from build123d import *

# Parameters (mm, degrees)
BOSS_EXTRUDE1_DEPTH = 50
BOSS_EXTRUDE2_DEPTH = 10
FILLET1_R           = 15
CUT_EXTRUDE1_START  = -3
CUT_EXTRUDE1_DEPTH  = 44
FILLET2_R           = 15
BOSS_EXTRUDE3_DEPTH = 50
SKETCH5_W           = 5.55555544444444
SKETCH5_H           = 7.560737598657919
SKETCH5_W_2         = 5.5555554444444475
SKETCH5_W_3         = 5.555555444444444
CUT_EXTRUDE2_DEPTH  = 68.02665161849878
CHAMFER1_SIZE       = 2.5
CHAMFER2_SIZE       = 1


with BuildPart() as part:
    # Sketch1 → Boss-Extrude1 (new body)
    with BuildSketch(Plane(origin=(0, 0, 0), x_dir=(0, 0, -1), z_dir=(1, 0, 0))):
        Polygon((0, 0), (50.00000000000001, 0), (16.66666666666667, -40), (-8.800000000000015, -17.499999999999996), (-8.800000000000015, -12.499999999999998), (-6.200000000000014, -12.499999999999998), (-6.200000000000013, -14.499999999999998), (-2.9999999999999982, -14.499999999999998), (-2.9999999999999982, -3), (-6.200000000000013, -3), (-6.200000000000014, -4.999999999999999), (-8.800000000000015, -4.999999999999999), (-8.800000000000017, -1.08e-15), align=None)
    extrude(amount=BOSS_EXTRUDE1_DEPTH)

    # Sketch2 → Boss-Extrude2 (add)
    with BuildSketch(Plane(origin=(50, 0, 0), x_dir=(0, 0, -1), z_dir=(1, 0, 0))):
        Polygon((-8.800000000000017, -1.08e-15), (-0.800000000000016, 0), (-0.8000000000000138, -17.499999999999996), (-8.800000000000015, -17.499999999999996), align=None)
    extrude(amount=-BOSS_EXTRUDE2_DEPTH)

    # Fillet1
    fillet1_edges = [part.edges().sort_by_distance(p)[0] for p in [
        (25, -40, -16.66666666666667),
    ]]
    fillet(fillet1_edges, radius=FILLET1_R)

    # Sketch3 → Cut-Extrude1 (cut)
    with BuildSketch(Plane(origin=(50, 0, 0), x_dir=(0, 0, -1), z_dir=(1, 0, 0)).offset(CUT_EXTRUDE1_START)):
        with BuildLine():
            Line((46.000000000000014, 0), (26.501646387603547, -23.398024334875757))
            add(Edge.make_bspline(
                [(0, -15), (11.33309259276565, -40.236961436031486), (26.501646387603547, -23.398024334875757)],
                knots=[0, 0, 0, 1, 1, 1], degree=2))
            Line((0, -15), (0, 0))
            Line((0, 0), (46.000000000000014, 0))
        make_face()
    extrude(amount=-CUT_EXTRUDE1_DEPTH, mode=Mode.SUBTRACT)

    # Fillet2
    fillet2_edges = [part.edges().sort_by_distance(p)[0] for p in [
        (25, -15, 0),
    ]]
    fillet(fillet2_edges, radius=FILLET2_R)

    # Sketch4 → Boss-Extrude3 (add, through all)
    with BuildSketch(Plane(origin=(50, 0, 0), x_dir=(0, 0, -1), z_dir=(1, 0, 0))):
        Polygon((50.00000000000001, 0), (46.000000000000014, 0), (49.20092199832241, 3.841106397986878), (53.20092199832241, 3.841106397986878), align=None)
    extrude(amount=-BOSS_EXTRUDE3_DEPTH)

    # Sketch5 → Cut-Extrude2 (cut, through all)
    with BuildSketch(Plane(origin=(0, -22.622950819672138, -27.147540983606568), x_dir=(1, 0, 0), z_dir=(0, 0.6401843996644799, 0.7682212795973757))):
        Polygon((11.111111, 29.44848238456608), (11.111111, 37.009219983224), (5.555555555555555, 37.009219983224), (5.555555555555556, 29.44848238456608), align=None)
        with Locations((19.444444277777777, 33.22885118389504)):
            Rectangle(SKETCH5_W, SKETCH5_H)
        with Locations((30.555555277777778, 33.22885118389504)):
            Rectangle(SKETCH5_W_2, SKETCH5_H)
        with Locations((41.66666627777778, 33.22885118389504)):
            Rectangle(SKETCH5_W_3, SKETCH5_H)
    extrude(amount=-CUT_EXTRUDE2_DEPTH, mode=Mode.SUBTRACT)

    # Chamfer1
    chamfer1_edges = [part.edges().sort_by_distance(p)[0] for p in [
        (8.333333277777777, -3.55e-15, -46.000000000000014),
        (19.444444277777777, -3.55e-15, -46.000000000000014),
        (30.555555277777778, -3.55e-15, -46.000000000000014),
        (41.66666627777778, -3.55e-15, -46.000000000000014),
    ]]
    chamfer(chamfer1_edges, length=CHAMFER1_SIZE)

    # Chamfer2
    chamfer2_edges = [part.edges().sort_by_distance(p)[0] for p in [
        (0, -12.499999999999998, 7.500000000000014),
        (0, -13.499999999999998, 6.2000000000000135),
        (0, -14.499999999999998, 4.600000000000005),
        (0, -8.75, 2.9999999999999982),
        (0, -3, 4.600000000000005),
        (0, -3.9999999999999996, 6.2000000000000135),
        (0, -4.999999999999999, 7.500000000000014),
    ]]
    chamfer(chamfer2_edges, length=CHAMFER2_SIZE)


solid = part.part
For this review, take the finished solid that the model builds, in its own axes (mm). A direction names the side the tool comes from. Round coordinates to 2 decimals unless told otherwise and drop trailing zeros. Loops run counter-clockwise (first coordinate to the right, second up) from the corner with the lowest first, then second, coordinate; pieces in that order, holes last. Notation, with made-up numbers: (38.25, 49) - (96.25, 49) arc R19 cw to (96.25, 54) - close; hole circle Ø8 at (87.5, -38.5). An arc over 180 degrees is marked (long way). Put each result on its own line as item: value. Start each with the question number.
1. Mouldability with a two-part tool opening along Y and no side actions: class faces 1 (the flat face through (30.52, -1.76, -46.18)), 2 (the flat face through (38.889, 1, -49)), 3 (the flat face through (25, -12, -40)), 4 (the flat face through (20, -3, 5)) as +Y half, -Y half, draft (parallel to the pull), parting line (faces both ways), or undercut.
2. For probe 1 along X at (y, z) = (-11.5, -9); probe 2 along Z at (x, y) = (36, -15.5); probe 3 along Z at (x, y) = (12, -17), list the stretches that pass through material, from the lowest coordinate up. Write a range as [from, to].
3. For faces 5 (the flat face through (36, 3.841, -51)), 6 (the flat face through (50, -15, -16)), 7 (the flat face through (20, -13, 6.2)), 8 (the flat face through (25.35, -9.97, -37.69)), 9 (the flat face through (20, -12.5, 8)), list the 3-axis set-ups (+Z, -Z, +X, -X, +Y, -Y) from which the entire face can be reached by the end or side of a thin tool; tool diameter is ignored.
4. Insertion check: P1, Ø4, axis at x = 29, y = -0.5, coming from the -Z side; P2, Ø3.5, axis at x = 23, z = 4, coming from the -Y side; P3, Ø2, axis at x = 11.5, y = -10.5, coming from the -Z side. Each pin has a flat end and moves straight along its axis. Give the tip position at first contact, or say it passes through.
5. Consider section A-A on z = -38.5. State the section outline as (x, y) points.
Result sheet:
1. face 1: +Y half
1. face 2: draft
1. face 3: -Y half
1. face 4: undercut
2. probe 1: [0, 3], [47, 50]
2. probe 2: [-37.08, -33.08], [-0.52, 8.8]
2. probe 3: [-35.83, -31.83], [-1.02, 8.8]
3. face 5: +Z, -Z, +X, -X, +Y
3. face 6: +Z, -Z, +X, +Y, -Y
3. face 7: -X
3. face 8: +Y
3. face 9: +Z, -X
4. P1: z = -50.9
4. P2: y = -23.29
4. P3: z = -42.08
5. outline: (0, -13.8) - (50, -13.8) - (50, 0) - (47, 0) - (47, -9) - (3, -9) - (3, 0) - (0, 0) - close
